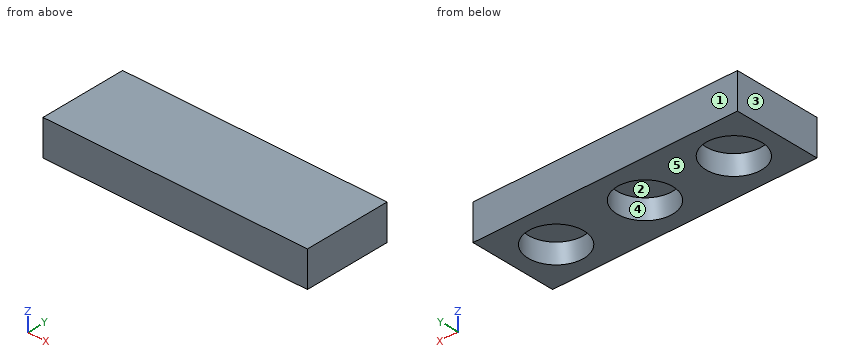
from build123d import *

# Parameters (mm, degrees)
SKETCH_1_W          = 23.8
SKETCH_1_H          = 7.8
EXTRUDE_1_DEPTH     = 3.2
SKETCH_2_R          = 2.5
CUT_EXTRUDE_1_DEPTH = 1.8


with BuildPart() as part:
    # Эскиз1 → Бобышка-Вытянуть1 (new body)
    with BuildSketch(Plane.XY):
        Rectangle(SKETCH_1_W, SKETCH_1_H)
    extrude(amount=EXTRUDE_1_DEPTH)

    # Эскиз2 → Вырез-Вытянуть1 (cut)
    with BuildSketch(Plane(origin=(0, 0, 0), x_dir=(-1, 0, 0), z_dir=(0, 0, -1))):
        Circle(SKETCH_2_R)
        with Locations((8, 0)):
            Circle(SKETCH_2_R)
        with Locations((-8, 0)):
            Circle(SKETCH_2_R)
    extrude(amount=-CUT_EXTRUDE_1_DEPTH, mode=Mode.SUBTRACT)


solid = part.part
Verification items for the finished model (mm, model axes). Face numbers are marked on the shaded views. A direction names the side the tool comes from. Give positions to 0.01 mm unless a question says otherwise; leave off trailing zeros. Write each loop counter-clockwise with the first axis right and the second up, starting at its lowest first coordinate (ties: lowest second). Pieces come first, ordered by that corner, then holes. Notation, with made-up numbers: M 70,-24.5 L 129,-24.5 A15 ccw 129,-9.5 Z; hole C 5,42.25 d1. An arc over 180 degrees is marked long. Put each result on its own line as item: value. Start each with the question number.
1. Section check A-A (z = 0.55). Record the cut outline in (x, y), and give its area (3 significant figures).
2. Section check B-B (y = 0). Record the cut outline in (x, z), and give its area (3 significant figures).
3. Scan lines: line 1 along Y through (x, z) = (8, 0.6); line 2 along X through (y, z) = (-0.5, 1.4); line 3 along X through (y, z) = (-1.75, 1.4). Record each from-to range of solid material in increasing order. Write a range as [from, to].
4. Go/stop test with a flat-tipped pin: pin 1 Ø1.5 at (x, y) = (0.5, 0.5) entering from -Z. Record where the tip stops, or that it passes through.
5. Draft check along Y on the marked faces 1, 2 and 3. Enter one of: +Y half, -Y half, draft (parallel to the pull), parting line (faces both ways), or undercut.
6. Set-up check for the marked faces 4 and 5: record each of +Z, -Z, +X, -X, +Y, -Y from which the full face is reachable in a straight line by a thin tool's end or side.
7. Section check D-D (x = 8). Record the cut outline in (y, z), and give its area (3 significant figures).
8. Section check C-C (x = 2). Record the cut outline in (y, z), and give its area (3 significant figures).
Answer list:
1. outline: M -11.9,-3.9 L 11.9,-3.9 L 11.9,3.9 L -11.9,3.9 Z; hole C -8,0 d5; hole C 0,0 d5; hole C 8,0 d5
1. area: 127 mm2
2. outline: M -11.9,0 L -10.5,0 L -10.5,1.8 L -5.5,1.8 L -5.5,0 L -2.5,0 L -2.5,1.8 L 2.5,1.8 L 2.5,0 L 5.5,0 L 5.5,1.8 L 10.5,1.8 L 10.5,0 L 11.9,0 L 11.9,3.2 L -11.9,3.2 Z
2. area: 49.2 mm2
3. line 1: [-3.9, -2.5], [2.5, 3.9]
3. line 2: [-11.9, -10.45], [-5.55, -2.45], [2.45, 5.55], [10.45, 11.9]
3. line 3: [-11.9, -9.79], [-6.21, -1.79], [1.79, 6.21], [9.79, 11.9]
4. pin 1: z = 1.8
5. face 1: +Y half
5. face 2: undercut
5. face 3: draft
6. face 4: -Z
6. face 5: -Z, +X, -X, +Y, -Y
7. outline: M -3.9,0 L -2.5,0 L -2.5,1.8 L 2.5,1.8 L 2.5,0 L 3.9,0 L 3.9,3.2 L -3.9,3.2 Z
7. area: 16.0 mm2
8. outline: M -3.9,0 L -1.5,0 L -1.5,1.8 L 1.5,1.8 L 1.5,0 L 3.9,0 L 3.9,3.2 L -3.9,3.2 Z
8. area: 19.6 mm2
